Design review of the part built by this model. Coordinates are the model's own, in mm. Face numbers are marked on the shaded views. A direction names the side the tool comes from. Give positions to 0.01 mm unless a question says otherwise; leave off trailing zeros. Order: outer loops, then holes, each group sorted by start corner. A loop starts at its lowest first (then second) coordinate and runs counter-clockwise, first axis right, second up. Notation, with made-up numbers: M 8,24 L 14,24 A13 ccw 14,33 Z; hole C 67,67 d6. An arc over 180 degrees is marked long. Answer as a JSON object with one key per item and string values.
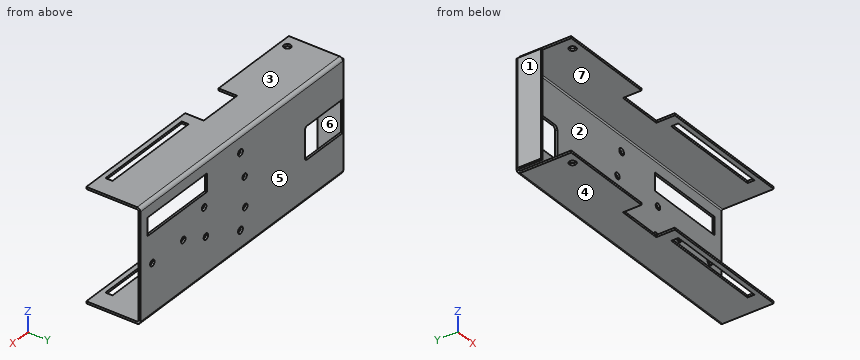
from build123d import *

# Parameters (mm, degrees)
SKETCH1_W          = 170
SKETCH1_H          = 65
BASE_FLANGE1_DEPTH = 1.29
EDGE_FLANGE1_DEPTH = 170
EDGE_FLANGE3_DEPTH = 65
CUT_EXTRUDE1_REACH = 187.022
SKETCH16_R         = 2
SKETCH16_W         = 50
SKETCH16_H         = 11
EDGE_FLANGE7_DEPTH = 170
SKETCH34_R         = 2.15
SKETCH34_W         = 28
SKETCH34_H         = 11.41
SKETCH34_W_2       = 64
SKETCH34_H_2       = 4.3
CUT_EXTRUDE5_DEPTH = 187.484767556
SKETCH36_R         = 1.875
CUT_EXTRUDE6_DEPTH = 10
SKETCH37_R         = 1.875
CUT_EXTRUDE7_DEPTH = 10


# Sheet-metal steps are written as plain solids
with BuildPart() as part:
    # Sketch1 → Base-Flange1 (new body)
    with BuildSketch(Plane(origin=(0, 0, 0), x_dir=(1, 0, 0), z_dir=(0, 1, 0))):
        with Locations((85, 32.5)):
            Rectangle(SKETCH1_W, SKETCH1_H)
    extrude(amount=-BASE_FLANGE1_DEPTH)

    # Edge-Flange1 section (across the edge) → Edge-Flange1 (add)
    with BuildSketch(Plane(origin=(170, -1.29, 0.7366), x_dir=(0, 0, -1), z_dir=(-1, 0, 0))):
        with BuildLine():
            Line((-1.29, 0.7366), (-1.29, 32))
            Line((-1.29, 32), (0, 32))
            Line((0, 32), (0, 0.7366))
            ThreePointArc((0, 0.7366), (0.215745145, 0.215745145), (0.7366, 0))
            Line((0.7366, 0), (0.7366, -1.29))
            ThreePointArc((0.7366, -1.29), (-0.696422603, -0.696422603), (-1.29, 0.7366))
        make_face()
    extrude(amount=EDGE_FLANGE1_DEPTH)

    # Edge-Flange3 section (across the edge) → Edge-Flange3 (add)
    with BuildSketch(Plane(origin=(-0.7366, -1.29, 0), x_dir=(1, 0, 0), z_dir=(0, 0, -1))):
        with BuildLine():
            Line((-1.29, 0.7366), (-1.29, 15))
            Line((-1.29, 15), (0, 15))
            Line((0, 15), (0, 0.7366))
            ThreePointArc((0, 0.7366), (0.215745145, 0.215745145), (0.7366, 0))
            Line((0.7366, 0), (0.7366, -1.29))
            ThreePointArc((0.7366, -1.29), (-0.696422603, -0.696422603), (-1.29, 0.7366))
        make_face()
    extrude(amount=EDGE_FLANGE3_DEPTH)

    # Sketch16 → Cut-Extrude1 (cut, up to next)
    with BuildSketch(Plane(origin=(0, 0, 0), x_dir=(1, 0, 0), z_dir=(0, 1, 0)), mode=Mode.PRIVATE) as cut_extrude1_sk1:
        with Locations(Location((86, 9, 0), (0, 0, 90))):
            Circle(SKETCH16_R)
    cut_extrude1_tool1 = extrude(cut_extrude1_sk1.sketch, amount=-CUT_EXTRUDE1_REACH, mode=Mode.PRIVATE) & part.part
    # Sketch16 → Cut-Extrude1 (cut, up to next)
    with BuildSketch(Plane(origin=(0, 0, 0), x_dir=(1, 0, 0), z_dir=(0, 1, 0)), mode=Mode.PRIVATE) as cut_extrude1_sk2:
        with Locations(Location((86, 55, 0), (0, 0, 90))):
            Circle(SKETCH16_R)
    cut_extrude1_tool2 = extrude(cut_extrude1_sk2.sketch, amount=-CUT_EXTRUDE1_REACH, mode=Mode.PRIVATE) & part.part
    # Sketch16 → Cut-Extrude1 (cut, up to next)
    with BuildSketch(Plane(origin=(0, 0, 0), x_dir=(1, 0, 0), z_dir=(0, 1, 0)), mode=Mode.PRIVATE) as cut_extrude1_sk3:
        with Locations((139, 12)):
            Rectangle(SKETCH16_W, SKETCH16_H)
    cut_extrude1_tool3 = extrude(cut_extrude1_sk3.sketch, amount=-CUT_EXTRUDE1_REACH, mode=Mode.PRIVATE) & part.part
    # Sketch16 → Cut-Extrude1 (cut, up to next)
    with BuildSketch(Plane(origin=(0, 0, 0), x_dir=(1, 0, 0), z_dir=(0, 1, 0)), mode=Mode.PRIVATE) as cut_extrude1_sk4:
        with BuildLine():
            Line((30, 42.5), (0, 42.5))
            Line((0, 42.5), (0, 22.5))
            Line((0, 22.5), (30, 22.5))
            ThreePointArc((30, 22.5), (31.414213562, 23.085786438), (32, 24.5))
            Line((32, 24.5), (32, 40.5))
            ThreePointArc((32, 40.5), (31.414213562, 41.914213562), (30, 42.5))
        make_face()
    cut_extrude1_tool4 = extrude(cut_extrude1_sk4.sketch, amount=-CUT_EXTRUDE1_REACH, mode=Mode.PRIVATE) & part.part
    add(cut_extrude1_tool1.solids().sort_by_distance((86, 0, -9))[0], mode=Mode.SUBTRACT)
    add(cut_extrude1_tool2.solids().sort_by_distance((86, 0, -55))[0], mode=Mode.SUBTRACT)
    add(cut_extrude1_tool3.solids().sort_by_distance((139, 0, -12))[0], mode=Mode.SUBTRACT)
    add(cut_extrude1_tool4.solids().sort_by_distance((15.958166, 0, -32.5))[0], mode=Mode.SUBTRACT)

    # Edge-Flange7 section (across the edge) → Edge-Flange7 (add)
    with BuildSketch(Plane(origin=(0, -1.29, -65.7366), x_dir=(0, 0, 1), z_dir=(1, 0, 0))):
        with BuildLine():
            Line((-1.29, 0.7366), (-1.29, 32))
            Line((-1.29, 32), (0, 32))
            Line((0, 32), (0, 0.7366))
            ThreePointArc((0, 0.7366), (0.215745145, 0.215745145), (0.7366, 0))
            Line((0.7366, 0), (0.7366, -1.29))
            ThreePointArc((0.7366, -1.29), (-0.696422603, -0.696422603), (-1.29, 0.7366))
        make_face()
    extrude(amount=EDGE_FLANGE7_DEPTH)

    # Sketch34 → Cut-Extrude5 (cut, through all)
    with BuildSketch(Plane(origin=(0, 0, -67.0266), x_dir=(-1, 0, 0), z_dir=(0, 0, -1))):
        with Locations(Location((-8, -28.29, 0), (0, 0, 270))):
            Circle(SKETCH34_R)
        with Locations((-73, -27.585)):
            Rectangle(SKETCH34_W, SKETCH34_H)
        with Locations((-126, -28.14)):
            Rectangle(SKETCH34_W_2, SKETCH34_H_2)
    extrude(amount=-CUT_EXTRUDE5_DEPTH, mode=Mode.SUBTRACT)

    # Sketch36 → Cut-Extrude6 (cut)
    with BuildSketch(Plane(origin=(0, 0, 0), x_dir=(1, 0, 0), z_dir=(0, 1, 0))):
        with Locations(Location((116.5, 25.5, 0), (0, 0, 270))):
            Circle(SKETCH36_R)
        with Locations(Location((115, 43.5, 0), (0, 0, 270))):
            Circle(SKETCH36_R)
        with Locations(Location((82.5, 25.1, 0), (0, 0, 270))):
            Circle(SKETCH36_R)
        with Locations(Location((82, 43.3, 0), (0, 0, 270))):
            Circle(SKETCH36_R)
    extrude(amount=-CUT_EXTRUDE6_DEPTH, mode=Mode.SUBTRACT)

    # Sketch37 → Cut-Extrude7 (cut)
    with BuildSketch(Plane(origin=(0, 0, 0), x_dir=(1, 0, 0), z_dir=(0, 1, 0))):
        with Locations(Location((160, 35.5, 0), (0, 0, 270))):
            Circle(SKETCH37_R)
        with Locations(Location((134, 35.5, 0), (0, 0, 270))):
            Circle(SKETCH37_R)
    extrude(amount=-CUT_EXTRUDE7_DEPTH, mode=Mode.SUBTRACT)


solid = part.part
(1) We need section A-A (x = 8). Write out the cut boundary in (y, z), plus the area to 3 significant figures.
Checked values:
{"outline": "M -33.29,-67.03 L -30.44,-67.03 L -30.44,-65.74 L -33.29,-65.74 Z; M -33.29,0.74 L -30.44,0.74 L -30.44,2.03 L -33.29,2.03 Z; M -26.14,-67.03 L -2.03,-67.03 A2.03 ccw 0,-65 L 0,-42.5 L -1.29,-42.5 L -1.29,-65 A0.74 cw -2.03,-65.74 L -26.14,-65.74 Z; M -26.14,0.74 L -2.03,0.74 A0.74 cw -1.29,0 L -1.29,-22.5 L 0,-22.5 L 0,0 A2.03 ccw -2.03,2.03 L -26.14,2.03 Z", "area": "133 mm^2"}
(2) Insertion check: pin 1 (0.6 mm diameter, centred on y = -0.5, z = -9.5, fed in from -X); pin 2 (0.6 mm diameter, centred on y = -12, z = 1.5, fed in from -X); pin 3 (0.6 mm diameter, centred on x = 128.5, y = -0.5, fed in from +Z); pin 4 (2 mm diameter, centred on x = 82.5, z = -25.1, fed in from -Y). Each pin has a flat end and moves straight along its axis. Give the tip position at first contact, or say it passes through.
Checked values:
{"pin 1": "stops at x = -1.61", "pin 2": "stops at x = 0", "pin 3": "stops at z = 1.61", "pin 4": "passes through"}
(3) We need section D-D (x = 66). Write out the cut boundary in (y, z).
Checked values:
{"outline": "M -21.88,-67.03 L -2.03,-67.03 A2.03 ccw 0,-65 L 0,0 A2.03 ccw -2.03,2.03 L -21.88,2.03 L -21.88,0.74 L -2.03,0.74 A0.74 cw -1.29,0 L -1.29,-65 A0.74 cw -2.03,-65.74 L -21.88,-65.74 Z"}
(4) To check wall thickness, follow L1, parallel to X at y = -28, z = -66; L2, parallel to Z at x = 97, y = -5; L3, parallel to X at y = -0.65, z = -25.5 (3 decimals). State the ranges of each line that lie inside material, in increasing order. Write a range as from..to.
Checked values:
{"L1": "x = 0..5.87, 10.13..59, 87..94, 158..170", "L2": "z = -67.03..-65.74, 0.74..2.03", "L3": "x = -1.487..0, 32..80.668, 84.332..114.625, 118.375..170"}
(5) We need section B-B (y = -19). Write out the cut boundary in (x, z), plus the area to 3 significant figures.
Checked values:
{"outline": "M 0,-67.03 L 170,-67.03 L 170,-65.74 L 0,-65.74 Z; M 0,0.74 L 170,0.74 L 170,2.03 L 0,2.03 Z", "area": "439 mm^2"}
(6) Tool access review of the marked faces 5, 6 and 7: name each direction out of +Z, -Z, +X, -X, +Y, -Y from which nothing blocks a thin tool from reaching the whole face with its end or side.
Checked values:
{"face 5": "+Z, -Z, +X, -X, +Y", "face 6": "+Z, -Z, +X, -Y", "face 7": "+X, -X, -Y"}
(7) Draft analysis for pull direction Z (two halves, no side actions). For the marked faces 1, 2, 3 and 4, state which applies: +Z half, -Z half, draft (parallel to the pull), parting line (faces both ways), or undercut.
Checked values:
{"face 1": "draft", "face 2": "undercut", "face 3": "+Z half", "face 4": "-Z half"}
(8) We need section C-C (z = -19.5). Write out the cut boundary in (x, y).
Checked values:
{"outline": "M -2.03,-16.29 L -0.74,-16.29 L -0.74,-2.03 A0.74 cw 0,-1.29 L 170,-1.29 L 170,0 L 0,0 A2.03 ccw -2.03,-2.03 Z"}
